Read the model definition and answer for the solid it produces. Units are mm, in the model's axes. Coordinates: 2 decimals unless noted, no trailing zeros. Order: outer loops, then holes, each group sorted by start corner. A loop starts at its lowest first (then second) coordinate and runs counter-clockwise, first axis right, second up. Notation, with made-up numbers: (28.25, 40.5) - (51.25, 40.5) arc R24 ccw to (51.25, 78.5) - close; hole circle Ø2 at (-15, 29.5). An arc over 180 degrees is marked (long way). Use one line per item in the form item = value.
```python
from build123d import *

# Parameters (mm, degrees)
F1_DEPTH = 101.6
F2_R     = 6.35
F3_DEPTH = 101.601


with BuildPart() as f1:
    # F0 (on Top) → F1 (new body)
    with BuildSketch(Plane.XY):
        with BuildLine():
            Line((0, 55.88), (-196.6468, 55.88))
            ThreePointArc((-196.6468, 55.88), (-252.5268, 0), (-196.6468, -55.88))
            Line((-196.6468, -55.88), (0, -55.88))
            ThreePointArc((0, -55.88), (55.88, 0), (0, 55.88))
        make_face()
    extrude(amount=F1_DEPTH)

    # F2 (on face) → F3 (cut, through all)
    with BuildSketch(Plane.XY.offset(101.6)):
        with Locations((-196.6468, 55.88)):
            Circle(F2_R)
        with Locations((-178.6128, 55.88)):
            Circle(F2_R)
        with Locations((-160.5788, 55.88)):
            Circle(F2_R)
        with Locations((-142.5448, 55.88)):
            Circle(F2_R)
        with Locations((-124.5108, 55.88)):
            Circle(F2_R)
        with Locations((-106.4768, 55.88)):
            Circle(F2_R)
        with Locations((-88.4428, 55.88)):
            Circle(F2_R)
        with Locations((-70.4088, 55.88)):
            Circle(F2_R)
        with Locations((-52.3748, 55.88)):
            Circle(F2_R)
        with Locations((-34.3408, 55.88)):
            Circle(F2_R)
        with Locations((-16.3068, 55.88)):
            Circle(F2_R)
        with Locations((1.7272, 55.88)):
            Circle(F2_R)
        with Locations((-196.6468, -55.88)):
            Circle(F2_R)
        with Locations((-178.6128, -55.88)):
            Circle(F2_R)
        with Locations((-160.5788, -55.88)):
            Circle(F2_R)
        with Locations((-142.5448, -55.88)):
            Circle(F2_R)
        with Locations((-124.5108, -55.88)):
            Circle(F2_R)
        with Locations((-106.4768, -55.88)):
            Circle(F2_R)
        with Locations((-88.4428, -55.88)):
            Circle(F2_R)
        with Locations((-70.4088, -55.88)):
            Circle(F2_R)
        with Locations((-52.3748, -55.88)):
            Circle(F2_R)
        with Locations((-34.3408, -55.88)):
            Circle(F2_R)
        with Locations((-16.3068, -55.88)):
            Circle(F2_R)
        with BuildLine():
            ThreePointArc((1.081132, -49.562952), (-2.528383, -60.593016), (8.0772, -55.88))
            ThreePointArc((8.0772, -55.88), (5.982783, -51.166984), (1.081132, -49.562952))
        make_face()
        with Locations((-215.758886, 52.510024)):
            Circle(F2_R)
        with Locations((-232.565772, 42.806563)):
            Circle(F2_R)
        with Locations((-245.0403, 27.94)):
            Circle(F2_R)
        with Locations((-251.677857, 9.70346)):
            Circle(F2_R)
        with Locations((-251.677857, -9.70346)):
            Circle(F2_R)
        with Locations((-245.0403, -27.94)):
            Circle(F2_R)
        with Locations((-232.565772, -42.806563)):
            Circle(F2_R)
        with Locations((-215.758886, -52.510024)):
            Circle(F2_R)
        with Locations((20.483246, 52.019172)):
            Circle(F2_R)
        with Locations((36.836167, 42.055374)):
            Circle(F2_R)
        with Locations((48.867411, 27.157574)):
            Circle(F2_R)
        with Locations((55.165454, 9.073605)):
            Circle(F2_R)
        with Locations((54.991401, -10.074893)):
            Circle(F2_R)
        with Locations((48.365671, -28.041389)):
            Circle(F2_R)
        with Locations((36.065606, -42.718026)):
            Circle(F2_R)
        with Locations((19.534267, -52.382917)):
            Circle(F2_R)
    extrude(amount=-F3_DEPTH, mode=Mode.SUBTRACT)


solid = f1.part
```
(1) Section B-B, the plane y = 27.94 is taken. Write down the section's boundary in (x, z).
Answer list:
outline = (-238.69, 0) - (42.57, 0) - (42.57, 101.6) - (-238.69, 101.6) - close
(2) Straight lines are drawn through the part: L1, parallel to X at y = 47, z = 44.5; L2, parallel to X at y = -47.5, z = 53.5; L3, parallel to X at y = -43.5, z = 15. For each, find the intervals that lie inside material, in ascending order.
Answer list:
L1 = -226.87 to -218.92, -212.6 to 16.59, 24.37 to 30.23
L2 = -226.08 to -219.66, -211.86 to 15.47, 23.59 to 29.43
L3 = -226.25 to 29.76
(3) Section A-A, the plane x = -197 is taken. Write down the section's boundary in (y, z), then the cut area to 3 significant figures.
Answer list:
outline = (-49.54, 0) - (49.54, 0) - (49.54, 101.6) - (-49.54, 101.6) - close
area = 10,100 mm2
(4) The mould has two halves that part along X. Classify faces 1 (the flat face through (-43, -55.88, 50)), 2 (the cylindrical face through (-206.3, 55.04, 50.09)), 3 (the cylindrical face through (52.8, 18.3, 50.1)), 4 (the cylindrical face through (-142.68, 49.53, 51.51)): +X half, -X half, draft (parallel to the pull), parting line (faces both ways), or undercut.
Answer list:
face_1 = draft
face_2 = -X half
face_3 = +X half
face_4 = undercut
(5) Given pin 1 Ø1.5 at (y, z) = (-43.5, 73) entering from +X; pin 2 Ø12 at (y, z) = (-3.5, 27.5) entering from +X; pin 3 Ø3 at (y, z) = (1.5, 83.5) entering from -X, each flat-ended and moving along its own axis, determine where each tip first touches the part or whether it passes through.
Answer list:
pin_1 = 29.9
pin_2 = 55.88
pin_3 = -252.53
